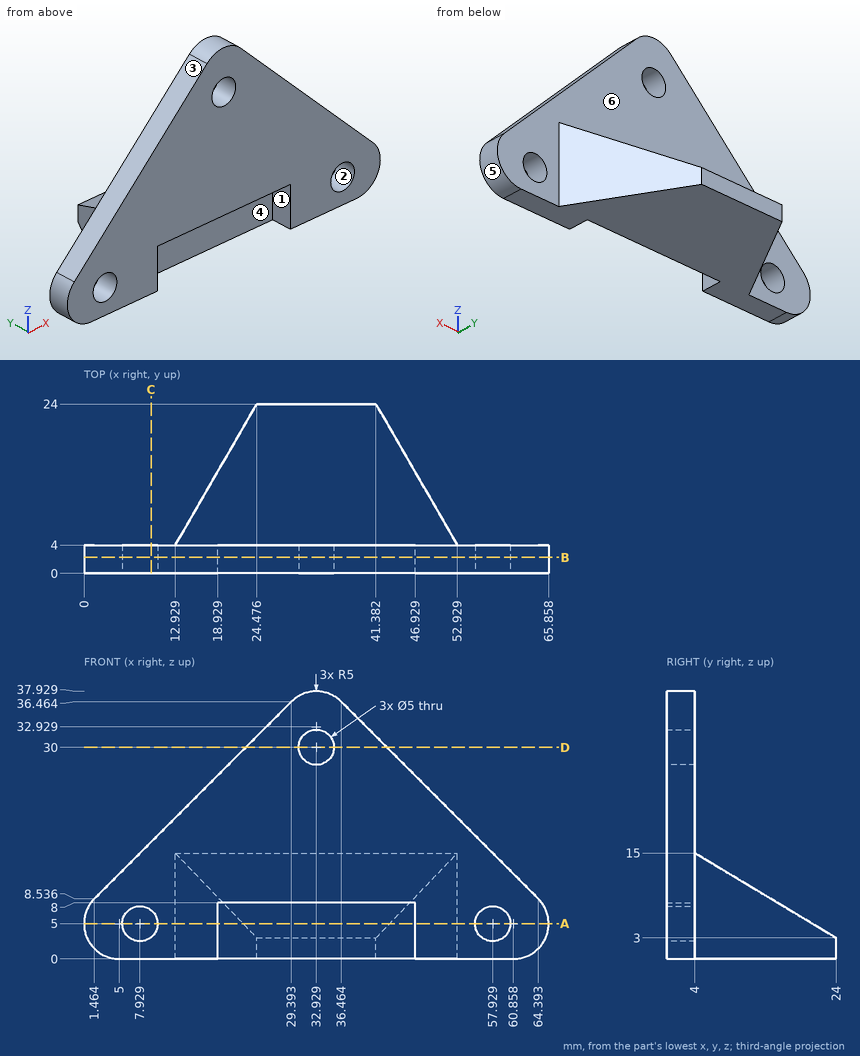
Geometry: see drawing. Coordinates: mm, zero at the bounding-box minimum. A direction names the side the tool comes from. Round coordinates to 2 decimals unless told otherwise and drop trailing zeros. Order: outer loops, then holes, each group sorted by start corner. A loop starts at its lowest first (then second) coordinate and runs counter-clockwise, first axis right, second up. Notation, with made-up numbers: (-34.75, 71) - (9.25, 71) arc R9 cw to (9.25, 76) - close; hole circle Ø9 at (-21.75, 76.5). An arc over 180 degrees is marked (long way). Use a Markdown table: item, result. Add a question column.
1. Line query: probe 1 along X at (y, z) = (1.8, 5); probe 2 along Y at (x, z) = (32.5, 33); probe 3 along X at (y, z) = (1.75, 30). Output: solid intervals per line, ascending.
2. Mould query, pull axis Z, two halves, no side actions, for the marked faces 1, 2 and 3. Classes: +Z half, -Z half, draft (parallel to the pull), parting line (faces both ways), or undercut.
3. Section query A-A (z = 5). Return the cut outline in (x, y), then the cut area to 3 significant figures.
4. First-contact query: pin 1 (8 mm diameter, centred on x = 20.5, z = 15.5, fed in from +Y) (1 decimal); pin 2 (1 mm diameter, centred on y = 3, z = 34, fed in from +X); pin 3 (2 mm diameter, centred on y = 6.5, z = 5, fed in from +X). Flat tips, straight axial feed; report the tip coordinate or a pass-through.
5. Section query C-C (x = 9.5). Return the cut outline in (y, z) (1 decimal).
6. Set-up query: the marked faces 4, 5 and 6. Return all of +Z, -Z, +X, -X, +Y, -Y with unobstructed straight access to the full face (end or side cutting, diameter ignored); none if empty.
7. Section query D-D (z = 30). Return the cut outline in (x, y).
8. Section query B-B (y = 2.25). Return the cut outline in (x, z) (1 decimal).
Derived:
| question | item | result |
|---|---|---|
| 1 | probe 1 | 0 to 5.43, 10.43 to 18.93, 46.93 to 55.43, 60.43 to 65.86 |
| 1 | probe 2 | 0 to 4 |
| 1 | probe 3 | 22.93 to 30.43, 35.43 to 42.93 |
| 2 | face 1 | draft |
| 2 | face 2 | undercut |
| 2 | face 3 | +Z half |
| 3 | outline | (0, 0) - (5.43, 0) - (5.43, 4) - (0, 4) - close; (10.43, 0) - (18.93, 0) - (18.93, 4) - (46.93, 4) - (46.93, 0) - (55.43, 0) - (55.43, 4) - (52.93, 4) - (43.31, 20.67) - (22.55, 20.67) - (12.93, 4) - (10.43, 4) - close; (60.43, 0) - (65.86, 0) - (65.86, 4) - (60.43, 4) - close |
| 3 | area | 618 mm2 |
| 4 | pin 1 | y = 9.8 |
| 4 | pin 2 | x = 39.43 |
| 4 | pin 3 | x = 52.06 |
| 5 | outline | (0, 0) - (4, 0) - (4, 3.1) - (0, 3.1) - close; (0, 6.9) - (4, 6.9) - (4, 16.6) - (0, 16.6) - close |
| 6 | face 4 | -Z, -Y |
| 6 | face 5 | +X, +Y, -Y |
| 6 | face 6 | +Z, +Y |
| 7 | outline | (22.93, 0) - (30.43, 0) - (30.43, 4) - (22.93, 4) - close; (35.43, 0) - (42.93, 0) - (42.93, 4) - (35.43, 4) - close |
| 8 | outline | (1.5, 8.5) arc R5 ccw to (5, 0) - (18.9, 0) - (18.9, 8) - (46.9, 8) - (46.9, 0) - (60.9, 0) arc R5 ccw to (64.4, 8.5) - (36.5, 36.5) arc R5 ccw to (29.4, 36.5) - close; hole circle Ø5 at (7.9, 5); hole circle Ø5 at (32.9, 30); hole circle Ø5 at (57.9, 5) |
